Study the drawing (mm; zero at the part's minimum x, y, z) and answer. A direction names the side the tool comes from. Round coordinates to 2 decimals unless told otherwise and drop trailing zeros. Loops run counter-clockwise (first coordinate to the right, second up) from the corner with the lowest first, then second, coordinate; pieces in that order, holes last. Notation, with made-up numbers: (-31, -9) - (-22, -9) arc R25 cw to (-22, 9) - close; hole circle Ø9 at (-23, 65.25). An arc over 180 degrees is marked (long way). Use CSV: the item, a comma, the result in double quotes. Start each with the question number.
1. Find section C-C (x = 3.75). Give the vertices of the cut face in (y, z).
2. Find section D-D (y = 7.5). Give the vertices of the cut face in (x, z).
3. A tool of negligible diameter and unlimited length cuts with its end or side. For the marked faces 1 and 2, from which of +Z, -Z, +X, -X, +Y, -Y can it reach the whole face along a straight path? Write none if from no direction.
4. Consider line 1 along X through (y, z) = (5, 5.5); line 2 along Y through (x, z) = (6.5, 5.5); line 3 along Y through (x, z) = (2, 3) (1 decimal). Determine where each line is inside the solid, lowest interval first.
5. Find section B-B (y = 4). Give the vertices of the cut face in (x, z), and give its area (3 significant figures).
6. Find section A-A (z = 1.25). Give the vertices of the cut face in (x, y), and give its area (3 significant figures).
7. Determine the mould class of the marked faces 3, 4 and 5 for opening direction X: +X half, -X half, draft (parallel to the pull), parting line (faces both ways), or undercut.
8. Given pin 1 Ø1 at (x, z) = (6, 4.5) entering from -Y; pin 2 Ø4 at (x, y) = (6, 3) entering from +Z; pin 3 Ø1 at (y, z) = (7, 2) entering from -X; pin 4 Ø2 at (y, z) = (7, 3) entering from +X (1 decimal), each flat-ended and moving along its own axis, determine where each tip first touches the part or whether it passes through.
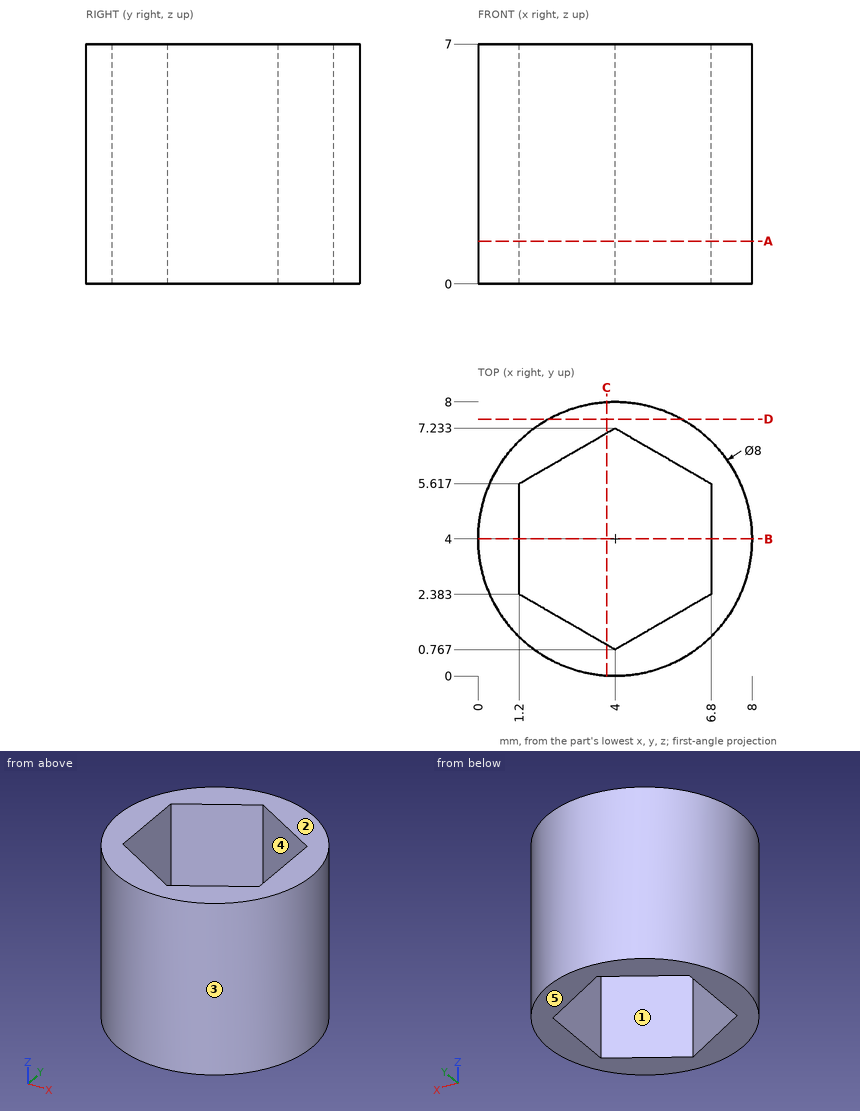
Filled sheet:
1,outline,"(0.01, 0) - (0.91, 0) - (0.91, 7) - (0.01, 7) - close; (7.09, 0) - (7.99, 0) - (7.99, 7) - (7.09, 7) - close"
2,outline,"(2.06, 0) - (5.94, 0) - (5.94, 7) - (2.06, 7) - close"
3,face 1,"+Z, -Z"
3,face 2,"+Z, +X, -X, +Y, -Y"
4,line 1,"x = 0.13 to 1.2, 6.8 to 7.87"
4,line 2,"y = 0.88 to 2.21, 5.79 to 7.12"
4,line 3,"y = 0.5 to 1.9, 6.1 to 7.5"
5,outline,"(0, 0) - (1.2, 0) - (1.2, 7) - (0, 7) - close; (6.8, 0) - (8, 0) - (8, 7) - (6.8, 7) - close"
5,area,"16.8 mm²"
6,outline,"circle Ø8 at (4, 4); hole (1.2, 2.38) - (4, 0.77) - (6.8, 2.38) - (6.8, 5.62) - (4, 7.23) - (1.2, 5.62) - close"
6,area,"23.1 mm²"
7,face 3,"parting line"
7,face 4,"undercut"
7,face 5,"draft"
8,pin 1,"stops at y = 0.29"
8,pin 2,"stops at z = 7"
8,pin 3,"stops at x = 0.88"
8,pin 4,"stops at x = 7.5"
